from build123d import *

# Parameters (mm, degrees)
F0_R     = 10.75
F1_DEPTH = 5.8
F2_R     = 4.75
F3_DEPTH = 2
F4_R     = 3
F5_DEPTH = 50.2
F6_R     = 3
F7_DEPTH = 5.2
F8_SIZE  = 0.5
F9_SIZE  = 0.2


with BuildPart() as f1:
    # F0 (on Front) → F1 (new body)
    with BuildSketch(Plane.XZ):
        Circle(F0_R)
    extrude(amount=F1_DEPTH)

    # F2 (on face) → F3 (join)
    with BuildSketch(Plane.XZ.offset(5.8)):
        Circle(F2_R)
    extrude(amount=F3_DEPTH)

    # F4 (on face) → F5 (join)
    with BuildSketch(Plane.XZ.offset(7.8)):
        Circle(F4_R)
    extrude(amount=F5_DEPTH)

    # F6 (on face) → F7 (join)
    with BuildSketch(Plane(origin=(0, 0, 0), x_dir=(-1, 0, 0), z_dir=(0, 1, 0))):
        Circle(F6_R)
    extrude(amount=F7_DEPTH)

    # F8
    f8_edges = [f1.edges().sort_by_distance(p)[0] for p in [
        (-10.75, -5.8, 0),
    ]]
    chamfer(f8_edges, length=F8_SIZE)

    # F9
    f9_edges = [f1.edges().sort_by_distance(p)[0] for p in [
        (-4.75, -7.8, 0),
        (-3, -58, 0),
        (3, 5.2, 0),
        (-10.75, 0, 0),
    ]]
    chamfer(f9_edges, length=F9_SIZE)


solid = f1.part
Can you work these out from the model? Positions are in its coordinate system, mm. A direction names the side the tool comes from. Give positions to 0.01 mm unless a question says otherwise; leave off trailing zeros. Loops run counter-clockwise (first coordinate to the right, second up) from the corner with the lowest first, then second, coordinate; pieces in that order, holes last. Notation, with made-up numbers: (85, 60.5) -> (134, 60.5) arc R20 ccw to (134, 85.5) -> close; hole circle Ø10 at (14, 30). An arc over 180 degrees is marked (long way). Use one line per item in the form item = value.
1) If we section it at B-B (x = 0): Please give me the cut outline in (y, z), plus the area to 3 significant figures.
Answers:
outline = (-58, -2.8) -> (-57.8, -3) -> (-7.8, -3) -> (-7.8, -4.55) -> (-7.6, -4.75) -> (-5.8, -4.75) -> (-5.8, -10.25) -> (-5.3, -10.75) -> (-0.2, -10.75) -> (0, -10.55) -> (0, -3) -> (5, -3) -> (5.2, -2.8) -> (5.2, 2.8) -> (5, 3) -> (0, 3) -> (0, 10.55) -> (-0.2, 10.75) -> (-5.3, 10.75) -> (-5.8, 10.25) -> (-5.8, 4.75) -> (-7.6, 4.75) -> (-7.8, 4.55) -> (-7.8, 3) -> (-57.8, 3) -> (-58, 2.8) -> close
area = 476 mm²
2) If we section it at A-A (z = 0): Please give me the cut outline in (x, y), plus the area to 3 significant figures.
Answers:
outline = (-10.75, -5.3) -> (-10.25, -5.8) -> (-4.75, -5.8) -> (-4.75, -7.6) -> (-4.55, -7.8) -> (-3, -7.8) -> (-3, -57.8) -> (-2.8, -58) -> (2.8, -58) -> (3, -57.8) -> (3, -7.8) -> (4.55, -7.8) -> (4.75, -7.6) -> (4.75, -5.8) -> (10.25, -5.8) -> (10.75, -5.3) -> (10.75, -0.2) -> (10.55, 0) -> (3, 0) -> (3, 5) -> (2.8, 5.2) -> (-2.8, 5.2) -> (-3, 5) -> (-3, 0) -> (-10.55, 0) -> (-10.75, -0.2) -> close
area = 476 mm²
3) If we section it at C-C (y = -1): Please give me the cut outline in (x, z), plus the area to 3 significant figures.
Answers:
outline = circle Ø21.5 at (0, 0)
area = 363 mm²
4) For faces 1 (the face through (-3, -32, 0)), 2 (the face through (0, 5.2, 0)), 3 (the face through (2.2, 0, 2.5)), which set-ups out of +Z, -Z, +X, -X, +Y, -Y let a thin tool reach every point of the face, with its end or its side?
Answers:
face_1 = -Y
face_2 = +Z, -Z, +X, -X, +Y
face_3 = +Y
5) If we section it at D-D (y = -9): Please give me the cut outline in (x, z).
Answers:
outline = circle Ø6 at (0, 0)
6) Will these pins go through, and if not, where does the flat tip stop? pin 1 (4 mm diameter, centred on x = 2.5, z = -6.5, fed in from +Y); pin 2 (8 mm diameter, centred on x = 6.5, y = -22, fed in from +Z); pin 3 (2 mm diameter, centred on x = 3.5, y = -14.5, fed in from -Z).
Answers:
pin_1 = 0
pin_2 = 1.66
pin_3 = -1.66
7) I need wall thicknesses on line 1 along Y through (x, z) = (-5.5, -8); line 2 along Y through (x, z) = (-1, 3); line 3 along Z through (x, y) = (0.5, -20.5). Which ranges of each line are inside material? Lowest first, please.
Answers:
line_1 = -5.8 to 0
line_2 = -7.8 to 0
line_3 = -2.96 to 2.96
